Autodesk Inventor part; units mm, degrees
ref_plane "YZ Plane" through (0, 0, 0) normal (1, 0, 0) x (0, 1, 0)
ref_plane "XZ Plane" through (0, 0, 0) normal (0, 1, 0) x (-1, 0, 0)
ref_plane "XY Plane" through (0, 0, 0) normal (0, 0, 1) x (1, 0, 0)
sketch "Sketch1" plane through (0, 0, 0) normal (0, 1, 0) x (-1, 0, 0)
  line L0 (10.5287, -10.7178) -> (-10.5287, -10.7178)
  line L1 (-10.5287, -10.7178) -> (-10.5287, 10.7178)
  line L2 (-10.5287, 10.7178) -> (10.5287, 10.7178)
  line L3 (10.5287, 10.7178) -> (10.5287, -10.7178)
  line L4 (10.5287, -10.7178) -> (-10.5287, 10.7178) construction
  line L5 (-10.5287, -10.7178) -> (10.5287, 10.7178) construction
  point P0 (0, 0)
extrude "Extrusion1" add sketch "Sketch1" along normal blind 10
shell "Shell1" thickness 1 removed faces 1 at (-3.5096, 10, -3.5726)
properties part number "Midsurf - DiffThick"
Verification items for the finished model (mm, model axes). A direction names the side the tool comes from. Give positions to 0.01 mm unless a question says otherwise; leave off trailing zeros. Order: outer loops, then holes, each group sorted by start corner. A loop starts at its lowest first (then second) coordinate and runs counter-clockwise, first axis right, second up. Notation, with made-up numbers: M 1,43 L 33,43 A4 ccw 33,49 Z; hole C 76,42.5 d4. An arc over 180 degrees is marked long. Answer as a JSON object with one key per item and string values. Group by question number.
1) Cross-section at B-B (y = 9.25). Enter the section's corners in (x, z), then the cut area to 3 significant figures.
2) Cross-section at C-C (z = -7.5). Enter the section's corners in (x, y).
3) Scan lines: line 1 along Z through (x, y) = (-7.25, 7.25); line 2 along X through (y, z) = (4.75, 2.75); line 3 along Y through (x, z) = (1.5, -1.5). Record each from-to range of solid material in increasing order. Write a range as [from, to].
4) Depth check by flat-ended pin: pin 1 Ø12 at (x, z) = (-5.5, 0) entering from +Y; pin 2 Ø5 at (x, z) = (4, 1) entering from +Y. Enter the tip coordinate at first touch or a pass-through.
5) Cross-section at A-A (x = 5.5). Enter the section's corners in (y, z), then the cut area to 3 significant figures.
6) Access from +Z, -Z, +X, -X, +Y, -Y to the whole of each face (thin tool, end or side, straight path). Record for faces 1 (the face through (10, 10, 0)), 2 (the face through (0, 1, 0)).
Result sheet:
{
 "1": {"outline": "M -10.53,-10.72 L 10.53,-10.72 L 10.53,10.72 L -10.53,10.72 Z; hole M -9.53,-9.72 L 9.53,-9.72 L 9.53,9.72 L -9.53,9.72 Z", "area": "81.0 mm2"},
 "2": {"outline": "M -10.53,0 L 10.53,0 L 10.53,10 L 9.53,10 L 9.53,1 L -9.53,1 L -9.53,10 L -10.53,10 Z"},
 "3": {"line 1": "z = [-10.72, -9.72], [9.72, 10.72]", "line 2": "x = [-10.53, -9.53], [9.53, 10.53]", "line 3": "y = [0, 1]"},
 "4": {"pin 1": "stops at y = 10", "pin 2": "stops at y = 1"},
 "5": {"outline": "M 0,-10.72 L 10,-10.72 L 10,-9.72 L 1,-9.72 L 1,9.72 L 10,9.72 L 10,10.72 L 0,10.72 Z", "area": "39.4 mm2"},
 "6": {"face 1": "+Z, -Z, +X, -X, +Y", "face 2": "+Y"}
}
